Part model, mm, in its own coordinate system. A direction names the side the tool comes from. Coordinates: 2 decimals unless noted, no trailing zeros. Loops run counter-clockwise (first coordinate to the right, second up) from the corner with the lowest first, then second, coordinate; pieces in that order, holes last. Notation, with made-up numbers: M 30,86 L 73,86 A4 cw 73,90 Z; hole C 29.5,75 d11. An arc over 180 degrees is marked long. Answer as a JSON object with one key per item and string values. Group by question number.
1. Saw through at C-C on x = 13.5. Write the cut outline in (y, z).
2. Mould opens along X. For faces 1 (the face through (7, -5, 2.159)), 2 (the face through (-4.63, -14, 4)) say: released by +X, released by -X, zero draft, split by the parting line, or undercut.
3. 3-axis set-ups, long thin cutter, end or side, ignore diameter. For faces 3 (the face through (6, -18.103, 9)), 4 (the face through (7, -1, 5.334)): which of +Z, -Z, +X, -X, +Y, -Y reach the whole face in a straight line?
4. Saw through at D-D on y = 22.5. Write the cut outline in (x, z).
5. Saw through at A-A on y = 29. Write the cut outline in (x, z).
6. Drill centre lines: L1, parallel to Y at x = -1.5, z = 5; L2, parallel to Y at x = 24, z = 2.5; L3, parallel to X at y = -14, z = 3.25. Where is each one in solid material? Low to high.
7. Drop flat-ended pins along their axis: pin 1 Ø2.5 at (x, z) = (13, 3.5) entering from -Y; pin 2 Ø2.5 at (x, y) = (-9.39, -11.75) entering from -Z; pin 3 Ø2.5 at (x, y) = (12.5, 8) entering from -Z; pin 4 Ø5 at (x, y) = (22.36, 26.35) entering from +Z. Give the stop position or say it passes through.
8. Saw through at B-B on x = -13. Write the cut outline in (y, z), then the cut area to 3 significant figures.
Autodesk Inventor part; units mm, degrees
ref_plane "Work Plane1" through (-16.0653, -32.8267, -33.655) normal (0, 0, -1) x (0, 1, 0)
ref_plane "YZ Plane" through (0, 0, 0) normal (1, 0, 0) x (0, 1, 0)
ref_plane "XZ Plane" through (0, 0, 0) normal (0, 1, 0) x (-1, 0, 0)
sketch "Sketch1" plane through (0, 0, 0) normal (0, 0, 1) x (1, 0, 0)
  circle A0 centre (22.3624, 26.3473) radius 1.5875
  circle A1 centre (22.3624, -11.7527) radius 1.5875
  circle A2 centre (-9.3876, 26.3473) radius 1.5875
  circle A3 centre (-9.3876, -11.7527) radius 1.5875
  line L0 (28.7124, 32.6973) -> (-15.7376, 32.6973)
  line L1 (-15.7376, 32.6973) -> (-15.7376, -18.1027)
  line L2 (-15.7376, -18.1027) -> (28.7124, -18.1027)
  line L3 (28.7124, -18.1027) -> (28.7124, 32.6973)
  point P0 (-3.5123, 7.2973)
  dimension "d26" = 50.8
  dimension "d27" = 44.45
  dimension "d28" = 6.35
  dimension "d29" = 6.35
  dimension "d30" = 6.35
  dimension "d31" = 6.35
  dimension "d32" = 6.35
  dimension "d33" = 6.35
  dimension "d34" = 6.35
  dimension "d35" = 6.35
  dimension "d44" = 3.175
  dimension "d45" = 3.175
  dimension "d46" = 3.175
  dimension "d47" = 3.175
extrude "Extrusion1" add sketch "Sketch1" along normal blind 12.7
sketch "Sketch2" plane through (-15.7376, -18.1027, 0) normal (0, -1, 0) x (1, 0, 0)
  line L0 (11.1075, 69.4178) -> (11.1075, 0)
  line L1 (33.3375, 69.1638) -> (33.3375, 0)
  line L2 (11.1075, 0) -> (33.3375, 0)
  line L3 (0, 9.525) -> (44.45, 9.525)
  line L4 (11.1075, 0) -> (33.3375, 0)
  line L5 (33.3375, 0) -> (33.3375, 5.334)
  line L6 (33.3375, 5.334) -> (11.1075, 5.334)
  line L7 (11.1075, 5.334) -> (11.1075, 0)
  line L8 (0, 0) -> (44.45, 0)
  point P0 (15.875, 0)
  point P1 (11.1075, 5.334)
  dimension "d2" = 5.334
  dimension "d21" = 0
extrude "Extrusion2" cut sketch "Sketch2" against normal blind 76.2 contours L6 L1 L2 L0
ref_plane "Work Plane1" through (-16.0653, -32.8267, -33.655) normal (0, 0, -1) x (0, 1, 0)
sketch "Sketch3" plane through (17.5999, -18.1027, 5.334) normal (0, 0, -1) x (-1, 0, 0)
  line L0 (0, 0) -> (0, 50.8)
  line L1 (0, 36.068) -> (22.23, 36.068)
  line L2 (22.23, 36.068) -> (22.23, 38.608)
  line L3 (22.23, 38.608) -> (0, 38.608)
  line L4 (0, 38.608) -> (0, 36.068)
  line L5 (0, 50.8) -> (22.23, 50.8)
  line L6 (33.3375, 65.3946) -> (33.3375, 0)
  line L7 (0, 28.068) -> (22.23, 28.068)
  line L8 (22.23, 28.068) -> (22.23, 30.608)
  line L9 (22.23, 30.608) -> (0, 30.608)
  line L10 (0, 30.608) -> (0, 28.068)
  line L11 (0, 20.068) -> (22.23, 20.068)
  line L12 (22.23, 20.068) -> (22.23, 22.608)
  line L13 (22.23, 22.608) -> (0, 22.608)
  line L14 (0, 22.608) -> (0, 20.068)
  line L15 (0, 12.068) -> (22.23, 12.068)
  line L16 (22.23, 12.068) -> (22.23, 14.608)
  line L17 (22.23, 14.608) -> (0, 14.608)
  line L18 (0, 14.608) -> (0, 12.068)
  point P0 (17.5999, 18.1027)
  point P1 (0, 14.608)
  point P2 (0, 12.068)
  point P3 (0, 22.608)
  point P4 (0, 20.068)
  point P5 (0, 30.608)
  point P6 (0, 28.068)
  point P7 (0, 38.608)
  dimension "d6" = 12.192
  dimension "d7" = 2.54
  dimension "d10" = 8
extrude "Extrusion3" add sketch "Sketch3" along normal blind 5.334
sketch "Sketch4" plane through (0, 0, 0) normal (0, 0, -1) x (-1, 0, 0)
  line L0 (-17.5999, 12.5053) -> (4.6301, 12.5053)
  line L1 (4.6301, 12.5053) -> (4.6301, 17.9653)
  line L2 (4.6301, 17.9653) -> (-17.5999, 17.9653)
  line L3 (-17.5999, 12.5053) -> (-17.5999, 17.9653)
  line L4 (-17.5999, 4.5053) -> (4.6301, 4.5053)
  line L5 (4.6301, 4.5053) -> (4.6301, 9.9653)
  line L6 (4.6301, 9.9653) -> (-17.5999, 9.9653)
  line L7 (-17.5999, 4.5053) -> (-17.5999, 9.9653)
  line L8 (4.6301, 1.9653) -> (-17.5999, 1.9653)
  line L9 (-17.5999, -3.4947) -> (-17.5999, 1.9653)
  line L10 (-17.5999, -3.4947) -> (4.6301, -3.4947)
  line L11 (4.6301, -3.4947) -> (4.6301, 1.9653)
  line L12 (4.6301, 20.5053) -> (4.6301, 32.6973)
  line L13 (4.6301, 20.5053) -> (20.4326, 20.5053)
  line L14 (20.4326, 20.5053) -> (20.4326, 23.6803)
  line L15 (20.4326, 23.6803) -> (4.6301, 23.6803)
  line L16 (4.6301, 23.6803) -> (4.6301, 20.5053)
  line L17 (4.6301, -6.0347) -> (-17.5999, -6.0347)
  line L18 (4.6301, -6.0347) -> (18.5436, -6.0347)
  line L19 (18.5436, -6.0347) -> (18.5436, -9.2097)
  line L20 (18.5436, -9.2097) -> (4.6301, -9.2097)
  line L21 (4.6301, -9.2097) -> (4.6301, -6.0347)
  line L22 (4.6301, 12.5053) -> (4.6301, 17.9653)
  line L23 (4.6301, 17.9653) -> (23.203, 17.9653)
  line L24 (23.203, 17.9653) -> (23.203, 12.5053)
  line L25 (23.203, 12.5053) -> (4.6301, 12.5053)
  line L26 (4.6301, 12.5053) -> (4.6301, 17.9653)
  line L27 (4.6301, 9.9653) -> (4.6301, 4.5053)
  line L28 (4.6301, 9.9653) -> (22.3845, 9.9653)
  line L29 (22.3845, 9.9653) -> (22.3845, 4.5053)
  line L30 (22.3845, 4.5053) -> (4.6301, 4.5053)
  line L31 (4.6301, 4.5053) -> (4.6301, 9.9653)
  line L32 (4.6301, 1.9653) -> (4.6301, -3.4947)
  line L33 (4.6301, 1.9653) -> (21.9437, 1.9653)
  line L34 (21.9437, 1.9653) -> (21.9437, -3.4947)
  line L35 (21.9437, -3.4947) -> (4.6301, -3.4947)
  line L36 (4.6301, -3.4947) -> (4.6301, 1.9653)
  line L37 (-17.5999, 17.9653) -> (-33.0876, 17.9653)
  line L38 (-33.0876, 17.9653) -> (-33.0876, 12.5053)
  line L39 (-33.0876, 12.5053) -> (-17.5999, 12.5053)
  line L40 (-17.5999, 12.5053) -> (-17.5999, 17.9653)
  line L41 (-17.5999, 9.9653) -> (-34.7876, 9.9653)
  line L42 (-34.7876, 9.9653) -> (-34.7876, 4.5053)
  line L43 (-34.7876, 4.5053) -> (-17.5999, 4.5053)
  line L44 (-17.5999, 4.5053) -> (-17.5999, 9.9653)
  line L45 (-17.5999, 1.9653) -> (4.6301, 1.9653)
  line L46 (-17.5999, 1.9653) -> (-33.0876, 1.9653)
  line L47 (-33.0876, 1.9653) -> (-33.0876, -3.4947)
  line L48 (-33.0876, -3.4947) -> (-17.5999, -3.4947)
  line L49 (-17.5999, -3.4947) -> (-17.5999, 1.9653)
  line L50 (-17.5999, 20.5053) -> (-30.1912, 20.5053)
  line L51 (-30.1912, 20.5053) -> (-30.1912, 23.6803)
  line L52 (-30.1912, 23.6803) -> (-17.5999, 23.6803)
  line L53 (-17.5999, 23.6803) -> (-17.5999, 20.5053)
  line L54 (-17.5999, -6.0347) -> (-30.1912, -6.0347)
  line L55 (-30.1912, -6.0347) -> (-30.1912, -9.2097)
  line L56 (-30.1912, -9.2097) -> (-17.5999, -9.2097)
  line L57 (-17.5999, -9.2097) -> (-17.5999, -6.0347)
  point P0 (-17.5999, -3.4947)
  point P1 (4.6301, -3.4947)
  point P2 (-17.5999, 4.5053)
  point P3 (4.6301, 4.5053)
  point P4 (-17.5999, 12.5053)
  point P5 (4.6301, 12.5053)
  point P6 (4.6301, 23.6803)
  dimension "d40" = 3.175
  dimension "d41" = 3.175
  dimension "d42" = 3.175
  dimension "d43" = 3.175
extrude "Extrusion4" cut sketch "Sketch4" against normal blind 5.334 contours L39 L38 L37 L3 | L1 L23 L24 L25 | L43 L42 L41 L7 | L5 L28 L29 L30 | L33 L34 L35 L11 | L9 L48 L47 L46 | L12 L15 L14 L13 | L57 L56 L55 L54 | L18 L19 L20 L21 | L50 L51 L52 L53
sketch "Sketch5" plane through (0, 0, 0) normal (0, 0, -1) x (-1, 0, 0)
  line L0 (17.6982, 39.5282) -> (-30.6897, 39.5282)
  line L1 (-30.6897, 39.5282) -> (-30.6897, -19.7169)
  line L2 (-30.6897, -19.7169) -> (17.6982, -19.7169)
  line L3 (17.6982, -19.7169) -> (17.6982, 39.5282)
extrude "Extrusion5" cut sketch "Sketch5" against normal blind 2.159
properties part number "Belt Clamp"
Outcome:
{
 "1": {"outline": "M -18.1,5.33 L -6.03,5.33 L -6.03,2.16 L -3.49,2.16 L -3.49,5.33 L 1.97,5.33 L 1.97,2.16 L 4.51,2.16 L 4.51,5.33 L 9.97,5.33 L 9.97,2.16 L 12.51,2.16 L 12.51,5.33 L 17.97,5.33 L 17.97,2.16 L 20.51,2.16 L 20.51,5.33 L 32.7,5.33 L 32.7,12.7 L -18.1,12.7 Z"},
 "2": {"face 1": "zero draft", "face 2": "undercut"},
 "3": {"face 3": "+Z, -Z, +X, -X, -Y", "face 4": "-Z, +X, -X"},
 "4": {"outline": "M -15.74,5.33 L 28.71,5.33 L 28.71,12.7 L -15.74,12.7 Z"},
 "5": {"outline": "M -15.74,2.16 L -4.63,2.16 L -4.63,5.33 L 17.6,5.33 L 17.6,2.16 L 28.71,2.16 L 28.71,12.7 L -15.74,12.7 Z"},
 "6": {"L1": "y = -6.03 to -3.49, 1.97 to 4.51, 9.97 to 12.51, 17.97 to 20.51", "L2": "y = -18.1 to -9.21, -6.03 to -3.49, 1.97 to 4.51, 9.97 to 12.51, 17.97 to 20.51, 23.68 to 32.7", "L3": "x = -15.74 to -4.63, 17.6 to 28.71"},
 "7": {"pin 1": "stops at y = -6.03", "pin 2": "passes through", "pin 3": "stops at z = 5.33", "pin 4": "stops at z = 12.7"},
 "8": {"outline": "M -18.1,2.16 L -9.21,2.16 L -9.21,5.33 L -6.03,5.33 L -6.03,2.16 L -3.49,2.16 L -3.49,5.33 L 1.97,5.33 L 1.97,2.16 L 4.51,2.16 L 4.51,5.33 L 9.97,5.33 L 9.97,2.16 L 12.51,2.16 L 12.51,5.33 L 17.97,5.33 L 17.97,2.16 L 20.51,2.16 L 20.51,5.33 L 23.68,5.33 L 23.68,2.16 L 32.7,2.16 L 32.7,12.7 L -18.1,12.7 Z", "area": "463 mm²"}
}
